Design review of the part built by this model. Coordinates are the model's own, in mm. A direction names the side the tool comes from. Give positions to 0.01 mm unless a question says otherwise; leave off trailing zeros. Write each loop counter-clockwise with the first axis right and the second up, starting at its lowest first coordinate (ties: lowest second). Pieces come first, ordered by that corner, then holes. Notation, with made-up numbers: (7.5, -21) -> (19.5, -21) arc R27 cw to (19.5, -5) -> close; hole circle Ø4 at (13, 29). An arc over 180 degrees is marked (long way). Answer as a JSON object with one key per item and string values.
```python
from build123d import *

# Parameters (mm, degrees)
F0_R     = 6.35
F1_DEPTH = 12.7
F2_SIZE  = 1.27
F4_DEPTH = 1.27


with BuildPart() as f1:
    # F0 (on Front) → F1 (new body)
    with BuildSketch(Plane.XZ):
        Polygon((9.348744, 5.3975), (0, 10.795), (-9.348744, 5.3975), (-9.348744, -5.3975), (0, -10.795), (9.348744, -5.3975), align=None)
        Circle(F0_R, mode=Mode.SUBTRACT)
    extrude(amount=F1_DEPTH)

    # F2
    f2_edges = [f1.edges().sort_by_distance(p)[0] for p in [
        (4.674372, -12.7, 8.09625),
        (9.348744, -12.7, 0),
        (4.674372, -12.7, -8.09625),
        (-4.674372, -12.7, -8.09625),
        (-9.348744, -12.7, 0),
        (-4.674372, -12.7, 8.09625),
    ]]
    chamfer(f2_edges, length=F2_SIZE)

    # F3 (on face) → F4 (join)
    with BuildSketch(Plane(origin=(0, 0, 0), x_dir=(-1, 0, 0), z_dir=(0, 1, 0))):
        Polygon((9.983744, -5.764117), (9.983744, 5.764117), (0, 11.528235), (-9.983744, 5.764117), (-9.983744, -5.764117), (0, -11.528235), align=None)
        Polygon((-9.348744, -5.3975), (-9.348744, 5.3975), (0, 10.795), (9.348744, 5.3975), (9.348744, -5.3975), (0, -10.795), align=None, mode=Mode.SUBTRACT)
    extrude(amount=-F4_DEPTH)


solid = f1.part
```
(1) For line 1 along Y through (x, z) = (-5.5, -7.5); line 2 along Z through (x, y) = (3.5, -5.25); line 3 along X through (y, z) = (-6.5, -1.75), list the stretches that pass through material, from the lowest coordinate up.
Here are the results:
{"line 1": "y = -11.53 to 0", "line 2": "z = -8.77 to -5.3, 5.3 to 8.77", "line 3": "x = -9.35 to -6.1, 6.1 to 9.35"}
(2) We need section C-C, the plane x = 2. State the section outline as (y, z) points.
Here are the results:
{"outline": "(-12.7, -8.17) -> (-11.43, -9.64) -> (-1.27, -9.64) -> (-1.27, -10.37) -> (0, -10.37) -> (0, -6.03) -> (-12.7, -6.03) -> close; (-12.7, 6.03) -> (0, 6.03) -> (0, 10.37) -> (-1.27, 10.37) -> (-1.27, 9.64) -> (-11.43, 9.64) -> (-12.7, 8.17) -> close"}
(3) For faces 5 (the flat face through (-9.349, -6, 0)), 6 (the flat face through (-4.74, -6.28, -8.06)), 7 (the flat face through (-4.4, -1.27, -8.5)), 8 (the flat face through (9.349, -6, 0)), list the 3-axis set-ups (+Z, -Z, +X, -X, +Y, -Y) from which the entire face can be reached by the end or side of a thin tool; tool diameter is ignored.
Here are the results:
{"face 5": "+Z, -Z, -X, -Y", "face 6": "-Z, -X, -Y", "face 7": "-Y", "face 8": "+Z, -Z, +X, -Y"}
(4) The part is to be moulded in two halves that separate along Z. For faces 1 (the flat face through (-9.984, -1, 0)), 2 (the flat face through (4.609, -6.279, -8.134)), 3 (the flat face through (4.9, -0.6, 8.7)), 4 (the cylindrical face through (-1.38, -6.26, -6.2)), say which applies: +Z half, -Z half, draft (parallel to the pull), parting line (faces both ways), or undercut.
Here are the results:
{"face 1": "draft", "face 2": "-Z half", "face 3": "+Z half", "face 4": "undercut"}
(5) Clearance check with flat-ended pins moving along their axes: pin 1 (5 mm diameter, centred on y = -3.5, z = -2.5, fed in from -X); pin 2 (5 mm diameter, centred on y = -5, z = 2, fed in from +X); pin 3 (1.5 mm diameter, centred on x = -7, z = -8, fed in from -Y); pin 4 (11.5 mm diameter, centred on x = 0, z = 0, fed in from +Y) (1 decimal). State where each tip first meets the part, or that it passes through.
Here are the results:
{"pin 1": "stops at x = -9.98", "pin 2": "stops at x = 9.35", "pin 3": "stops at y = -1.27", "pin 4": "passes through"}
(6) We need section D-D, the plane x = 8.5. State the section outline as (y, z) points.
Here are the results:
{"outline": "(-12.28, -4.91) -> (-11.43, -5.89) -> (-1.27, -5.89) -> (-1.27, -6.62) -> (0, -6.62) -> (0, 6.62) -> (-1.27, 6.62) -> (-1.27, 5.89) -> (-11.43, 5.89) -> (-12.28, 4.91) -> close"}
(7) We need section A-A, the plane z = 0. State the section outline as (x, y) points.
Here are the results:
{"outline": "(-9.98, -1.27) -> (-9.35, -1.27) -> (-9.35, -11.43) -> (-8.08, -12.7) -> (-6.35, -12.7) -> (-6.35, 0) -> (-9.98, 0) -> close; (6.35, -12.7) -> (8.08, -12.7) -> (9.35, -11.43) -> (9.35, -1.27) -> (9.98, -1.27) -> (9.98, 0) -> (6.35, 0) -> close"}
